```python
from build123d import *

# Parameters (mm, degrees)
EXTRUDE_1_DEPTH = 5
EXTRUDE_START   = -15
EXTRUDE_2_DEPTH = 5
FILLET_1_R      = 3


with BuildPart() as part:
    # Эскиз1 → Бобышка-Вытянуть1 (new body)
    with BuildSketch(Plane.XY):
        with BuildLine():
            Line((-13.101757321, 110.493831222), (-13.101757321, 80.493831222))
            ThreePointArc((-13.101757321, 80.493831222), (-20.601757321, 72.993831222), (-28.101757321, 80.493831222))
            Line((-28.101757321, 80.493831222), (-28.101757321, 110.493831222))
            ThreePointArc((-28.101757321, 110.493831222), (-20.601757321, 117.993831222), (-13.101757321, 110.493831222))
        make_face()
    extrude(amount=EXTRUDE_1_DEPTH)

    # Эскиз2 → Бобышка-Вытянуть2 (add)
    with BuildSketch(Plane.ZY.offset(28.101757321).offset(EXTRUDE_START)):
        with BuildLine():
            Line((5, 103.493831222), (25, 103.493831222))
            ThreePointArc((25, 103.493831222), (33, 95.493831222), (25, 87.493831222))
            Line((25, 87.493831222), (5, 87.493831222))
            Line((5, 87.493831222), (5, 103.493831222))
        make_face()
        with BuildLine():
            Line((25, 93.993831222), (12, 93.993831222))
            ThreePointArc((12, 93.993831222), (10.5, 95.493831222), (12, 96.993831222))
            Line((12, 96.993831222), (25, 96.993831222))
            ThreePointArc((25, 96.993831222), (26.5, 95.493831222), (25, 93.993831222))
        make_face(mode=Mode.SUBTRACT)
    extrude(amount=EXTRUDE_2_DEPTH)

    # Скругление1
    fillet_1_edges = [part.edges().sort_by_distance(p)[0] for p in [
        (-18.101757321, 95.493831222, 5),
        (-15.601757321, 87.493831222, 5),
        (-15.601757321, 103.493831222, 5),
    ]]
    fillet(fillet_1_edges, radius=FILLET_1_R)


solid = part.part
```
Build history of the part. All positions in model axes, mm. A direction names the side the tool comes from. Coordinates: 2 decimals unless noted, no trailing zeros. Write each loop counter-clockwise with the first axis right and the second up, starting at its lowest first coordinate (ties: lowest second). Pieces come first, ordered by that corner, then holes.
1. Band-saw the part on D-D, the plane z = 4. Give the cut face in (x, y), and give its area (3 significant figures).
Answer block:
outline: (-28.1, 80.49) arc R7.5 ccw to (-13.1, 80.49) - (-13.1, 110.49) arc R7.5 ccw to (-28.1, 110.49) - close
area: 627 mm2
2. Band-saw the part on B-B, the plane x = -15. Give the cut face in (y, z).
Answer block:
outline: (75.51, 0) - (115.48, 0) - (115.48, 5) - (106.49, 5) arc R3 cw to (103.49, 8) - (103.49, 25) arc R8 ccw to (87.49, 25) - (87.49, 8) arc R3 cw to (84.49, 5) - (75.51, 5) - close; hole (93.99, 12) arc R1.5 ccw to (96.99, 12) - (96.99, 25) arc R1.5 ccw to (93.99, 25) - close
3. Drop flat-ended pins along their axis: pin 1 (8 mm diameter, centred on x = -20, y = 103, fed in from +Z); pin 2 (2.5 mm diameter, centred on x = -15, z = 17.5, fed in from -Y); pin 3 (8 mm diameter, centred on y = 92, z = 20.5, fed in from -X). Give the stop position or say it passes through.
Answer block:
pin 1: stops at z = 31.94
pin 2: stops at y = 87.49
pin 3: stops at x = -18.1
4. Band-saw the part on C-C, the plane y = 102.5. Give the cut face in (x, z), and give its area (3 significant figures).
Answer block:
outline: (-28.1, 0) - (-13.1, 0) - (-13.1, 28.86) - (-18.1, 28.86) - (-18.1, 8) arc R3 cw to (-21.1, 5) - (-28.1, 5) - close
area: 196 mm2
5. Band-saw the part on A-A, the plane z = 26. Give the cut face in (x, y).
Answer block:
outline: (-18.1, 87.56) - (-13.1, 87.56) - (-13.1, 94.38) - (-18.1, 94.38) - close; (-18.1, 96.61) - (-13.1, 96.61) - (-13.1, 103.43) - (-18.1, 103.43) - close
6. Pull direction Z, two halves, no side cores. Call faces 1 (the cylindrical face through (-20.437, 72.996, 2.465)), 2 (the cylindrical face through (-16.269, 104.396, 5.855)), 3 (the flat face through (-16, 93.994, 19)): released by +Z, released by -Z, zero draft, split by the parting line, or undercut.
Answer block:
face 1: zero draft
face 2: released by +Z
face 3: undercut
7. Drill centre lines: probe 1 along Z at (x, y) = (-23.5, 81); probe 2 along X at (y, z) = (91.5, 17.5); probe 3 along Y at (x, z) = (-14.5, 9.5). Where is each one in solid material? Low to high.
Answer block:
probe 1: z = 0 to 5
probe 2: x = -18.1 to -13.1
probe 3: y = 87.49 to 103.49
8. 3-axis set-ups, long thin cutter, end or side, ignore diameter. For faces 4 (the flat face through (-22, 96, 5)), 5 (the flat face through (-18.102, 97.4, 20.7)), 6 (the cylindrical face through (-15.6, 95.5, 26.5)): which of +Z, -Z, +X, -X, +Y, -Y reach the whole face in a straight line?
Answer block:
face 4: +Z, -X
face 5: +Z, -X, +Y, -Y
face 6: +X, -X
